Can you work these out from the model? Positions are in its coordinate system, mm. Face numbers are marked on the shaded views. Round coordinates to 2 decimals unless told otherwise and drop trailing zeros. Loops run counter-clockwise (first coordinate to the right, second up) from the corner with the lowest first, then second, coordinate; pieces in that order, holes last. Notation, with made-up numbers: (17, -4.75) -> (69, -4.75) arc R11 cw to (69, 2.25) -> close; hole circle Ø7 at (2, 38). An arc over 180 degrees is marked (long way). Write each question's results on one line, items separated by ' | '.
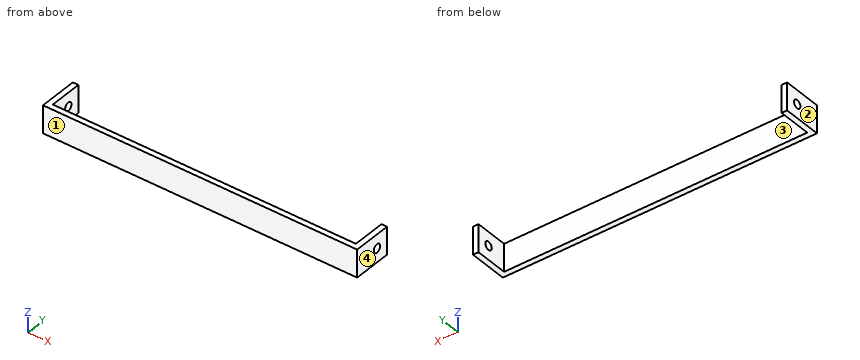
from build123d import *

# Parameters (mm, degrees)
BOSS_EXTRU_1_DEPTH           = 10
ENL_V_MAT_EXTRU_1_DEPTH      = 116.290936331
ENL_V_MAT_EXTRU_1_DEPTH_BACK = 116.290936331
ESQUISSE2_R                  = 1.5


with BuildPart() as part:
    # Esquisse1 → Boss.-Extru.1 (new body)
    with BuildSketch(Plane.XY):
        Polygon((57, 0), (-57, 0), (-57, 14), (-55, 14), (-55, 2), (55, 2), (55, 14), (57, 14), align=None)
    extrude(amount=BOSS_EXTRU_1_DEPTH)

    # Esquisse2 → Enlèv. mat.-Extru.1 (cut, two sides: drawn at the far end of the back side and taken through both)
    with BuildSketch(Plane.ZY.offset(57).offset(-ENL_V_MAT_EXTRU_1_DEPTH_BACK)):
        with Locations((5, 9.284897648)):
            Circle(ESQUISSE2_R)
    extrude(amount=ENL_V_MAT_EXTRU_1_DEPTH + ENL_V_MAT_EXTRU_1_DEPTH_BACK, mode=Mode.SUBTRACT)


solid = part.part
1. We'd pull the mould along X, two halves only. Please class the marked faces 1, 2, 3 and 4: pulls with the +X half, pulls with the -X half, needs draft (parallel to the pull), parting line crosses it, or undercut.
Final values:
face 1: needs draft | face 2: pulls with the -X half | face 3: undercut | face 4: pulls with the +X half
2. If we section it at C-C (x = 5.5): List the corners of the cut face in (y, z) for me, then the cut area to 3 significant figures.
Final values:
outline: (0, 0) -> (2, 0) -> (2, 10) -> (0, 10) -> close | area: 20.0 mm2
3. If we section it at B-B (y = 4.75): List the corners of the cut face in (x, z) for me, then the cut area to 3 significant figures.
Final values:
outline: (-57, 0) -> (-55, 0) -> (-55, 10) -> (-57, 10) -> close; (55, 0) -> (57, 0) -> (57, 10) -> (55, 10) -> close | area: 40.0 mm2
4. Please list where these lines run through material, in increasing order: line 1 (X direction, y = 8, z = 1); line 2 (Y direction, x = -55.7, z = 5); line 3 (Y direction, x = -27.5, z = 9). Write a range as from..to.
Final values:
line 1: -57..-55, 55..57 | line 2: 0..7.78, 10.78..14 | line 3: 0..2
5. If we section it at A-A (z = 5): List the corners of the cut face in (x, y) for me.
Final values:
outline: (-57, 0) -> (57, 0) -> (57, 7.78) -> (55, 7.78) -> (55, 2) -> (-55, 2) -> (-55, 7.78) -> (-57, 7.78) -> close; (-57, 10.78) -> (-55, 10.78) -> (-55, 14) -> (-57, 14) -> close; (55, 10.78) -> (57, 10.78) -> (57, 14) -> (55, 14) -> close
6. Will these pins go through, and if not, where does the flat tip stop? pin 1 (2.5 mm diameter, centred on y = 9.28, z = 5, fed in from -X); pin 2 (6 mm diameter, centred on x = -2, z = 7, fed in from +Y).
Final values:
pin 1: through | pin 2: y = 2
